```python
from build123d import *

# Parameters (mm, degrees)
F0_R     = 6.35
F1_DEPTH = 3.81


with BuildPart() as f1:
    # F0 (on Top) → F1 (new body, symmetric)
    with BuildSketch(Plane.XY):
        with BuildLine():
            Line((-22.269135, -16.838492), (-20.069431, -15.568492))
            ThreePointArc((-20.069431, -15.568492), (-17.960512, -17.960512), (-15.568492, -20.069431))
            Line((-15.568492, -20.069431), (-16.838492, -22.269135))
            Line((-16.838492, -22.269135), (-18.675675, -26.759218))
            Line((-18.675675, -26.759218), (-16.256, -28.156218))
            Line((-16.256, -28.156218), (-13.836325, -29.553218))
            Line((-13.836325, -29.553218), (-10.866391, -25.71713))
            Line((-10.866391, -25.71713), (-9.596391, -23.517425))
            ThreePointArc((-9.596391, -23.517425), (-6.574004, -24.534516), (-3.447994, -25.164883))
            Line((-3.447994, -25.164883), (-3.447994, -27.704883))
            Line((-3.447994, -27.704883), (-2.794, -32.512))
            Line((-2.794, -32.512), (0, -32.512))
            Line((0, -32.512), (2.794, -32.512))
            Line((2.794, -32.512), (3.447994, -27.704883))
            Line((3.447994, -27.704883), (3.447994, -25.164883))
            ThreePointArc((3.447994, -25.164883), (6.574004, -24.534516), (9.596391, -23.517425))
            Line((9.596391, -23.517425), (10.866391, -25.71713))
            Line((10.866391, -25.71713), (13.836325, -29.553218))
            Line((13.836325, -29.553218), (16.256, -28.156218))
            Line((16.256, -28.156218), (18.675675, -26.759218))
            Line((18.675675, -26.759218), (16.838492, -22.269135))
            Line((16.838492, -22.269135), (15.568492, -20.069431))
            ThreePointArc((15.568492, -20.069431), (17.960512, -17.960512), (20.069431, -15.568492))
            Line((20.069431, -15.568492), (22.269135, -16.838492))
            Line((22.269135, -16.838492), (26.759218, -18.675675))
            Line((26.759218, -18.675675), (28.156218, -16.256))
            Line((28.156218, -16.256), (29.553218, -13.836325))
            Line((29.553218, -13.836325), (25.71713, -10.866391))
            Line((25.71713, -10.866391), (23.517425, -9.596391))
            ThreePointArc((23.517425, -9.596391), (24.534516, -6.574004), (25.164883, -3.447994))
            ThreePointArc((25.164883, -3.447994), (25.4, 0), (25.164883, 3.447994))
            ThreePointArc((25.164883, 3.447994), (24.534516, 6.574004), (23.517425, 9.596391))
            ThreePointArc((23.517425, 9.596391), (21.997045, 12.7), (20.069431, 15.568492))
            ThreePointArc((20.069431, 15.568492), (17.960512, 17.960512), (15.568492, 20.069431))
            Line((15.568492, 20.069431), (16.838492, 22.269135))
            Line((16.838492, 22.269135), (18.675675, 26.759218))
            Line((18.675675, 26.759218), (16.256, 28.156218))
            Line((16.256, 28.156218), (13.836325, 29.553218))
            Line((13.836325, 29.553218), (10.866391, 25.71713))
            Line((10.866391, 25.71713), (9.596391, 23.517425))
            ThreePointArc((9.596391, 23.517425), (6.574004, 24.534516), (3.447994, 25.164883))
            Line((3.447994, 25.164883), (3.447994, 27.704883))
            Line((3.447994, 27.704883), (2.794, 32.512))
            Line((2.794, 32.512), (0, 32.512))
            Line((0, 32.512), (-2.794, 32.512))
            Line((-2.794, 32.512), (-3.447994, 27.704883))
            Line((-3.447994, 27.704883), (-3.447994, 25.164883))
            ThreePointArc((-3.447994, 25.164883), (-6.574004, 24.534516), (-9.596391, 23.517425))
            Line((-9.596391, 23.517425), (-10.866391, 25.71713))
            Line((-10.866391, 25.71713), (-13.836325, 29.553218))
            Line((-13.836325, 29.553218), (-16.256, 28.156218))
            Line((-16.256, 28.156218), (-18.675675, 26.759218))
            Line((-18.675675, 26.759218), (-16.838492, 22.269135))
            Line((-16.838492, 22.269135), (-15.568492, 20.069431))
            ThreePointArc((-15.568492, 20.069431), (-17.960512, 17.960512), (-20.069431, 15.568492))
            Line((-20.069431, 15.568492), (-22.269135, 16.838492))
            Line((-22.269135, 16.838492), (-26.759218, 18.675675))
            Line((-26.759218, 18.675675), (-28.156218, 16.256))
            Line((-28.156218, 16.256), (-29.553218, 13.836325))
            Line((-29.553218, 13.836325), (-25.71713, 10.866391))
            Line((-25.71713, 10.866391), (-23.517425, 9.596391))
            ThreePointArc((-23.517425, 9.596391), (-24.534516, 6.574004), (-25.164883, 3.447994))
            Line((-25.164883, 3.447994), (-27.704883, 3.447994))
            Line((-27.704883, 3.447994), (-32.512, 2.794))
            Line((-32.512, 2.794), (-32.512, 0))
            Line((-32.512, 0), (-32.512, -2.794))
            Line((-32.512, -2.794), (-27.704883, -3.447994))
            Line((-27.704883, -3.447994), (-25.164883, -3.447994))
            ThreePointArc((-25.164883, -3.447994), (-24.534516, -6.574004), (-23.517425, -9.596391))
            Line((-23.517425, -9.596391), (-25.71713, -10.866391))
            Line((-25.71713, -10.866391), (-29.553218, -13.836325))
            Line((-29.553218, -13.836325), (-28.156218, -16.256))
            Line((-28.156218, -16.256), (-26.759218, -18.675675))
            Line((-26.759218, -18.675675), (-22.269135, -16.838492))
        make_face()
        Circle(F0_R, mode=Mode.SUBTRACT)
    extrude(amount=F1_DEPTH, both=True)


solid = f1.part
```
Check sheet for the modelled part. Datum: model origin and axes. Units: mm. A direction names the side the tool comes from. Coordinates: 2 decimals unless noted, no trailing zeros. Order: outer loops, then holes, each group sorted by start corner. A loop starts at its lowest first (then second) coordinate and runs counter-clockwise, first axis right, second up. Notation, with made-up numbers: (84, 62.5) -> (139, 62.5) arc R20 cw to (139, 94.5) -> close; hole circle Ø10 at (41.5, 50.25). An arc over 180 degrees is marked (long way). Write item = value, one per line. Start each with the question number.
1) Cross-section at B-B (x = 0). Enter the section's corners in (y, z).
2) Cross-section at C-C (x = 7.5). Enter the section's corners in (y, z).
3) Cross-section at A-A (y = 0). Enter the section's corners in (x, z), then the cut area to 3 significant figures.
4) Access from +Z, -Z, +X, -X, +Y, -Y to the whole of each face (thin tool, end or side, straight path). Record for faces 1 (the flat face through (-3.126, -30.075, 0.053)), 2 (the cylindrical face through (24.546, 6.531, 0.053)), 3 (the flat face through (-24.6, -10.22, 0.05)), 4 (the flat face through (-32.512, 0, 0)), 5 (the flat face through (-10.22, 24.6, 0.05)).
5) Material ranges on L1, parallel to Y at x = 0, z = 1.25; L2, parallel to Y at x = -17.5, z = -1.5; L3, parallel to Y at x = -18.5, z = -2.5, recorded low to high.
6) Mould release check, pull along Y, two halves, no side actions. Record for faces 6 (the flat face through (-26, 3.448, 0)), 7 (the flat face through (3.116, -30.142, 0.053)), 8 (the flat face through (0, 32.512, 0)), 9 (the flat face through (-2, -7, -3.81)): +Y half, -Y half, draft (parallel to the pull), parting line (faces both ways), or undercut.
7) Go/stop test with flat-tipped pins: P1, Ø3, axis at x = -13.5, z = -1, coming from the +Y side; P2, Ø2, axis at y = -24, z = 1.5, coming from the +X side; P3, Ø0.8, axis at x = -26, z = 1.5, coming from the +Y side. Record where each tip stops, or that it passes through.
Ans:
q1.outline = (-32.51, -3.81) -> (-6.35, -3.81) -> (-6.35, 3.81) -> (-32.51, 3.81) -> close; (6.35, -3.81) -> (32.51, -3.81) -> (32.51, 3.81) -> (6.35, 3.81) -> close
q2.outline = (-24.27, -3.81) -> (24.27, -3.81) -> (24.27, 3.81) -> (-24.27, 3.81) -> close
q3.outline = (-32.51, -3.81) -> (-6.35, -3.81) -> (-6.35, 3.81) -> (-32.51, 3.81) -> close; (6.35, -3.81) -> (25.4, -3.81) -> (25.4, 3.81) -> (6.35, 3.81) -> close
q3.area = 345 mm²
q4.face_1 = +Z, -Z, -Y
q4.face_2 = +Z, -Z, +X, +Y
q4.face_3 = +Z, -Z, -X
q4.face_4 = +Z, -Z, -X, +Y, -Y
q4.face_5 = +Z, -Z, +Y
q5.L1 = -32.51 to -6.35, 6.35 to 32.51
q5.L2 = -27.44 to -23.89, -18.41 to 18.41, 23.89 to 27.44
q5.L3 = -26.86 to -26.33, -17.4 to 17.4, 26.33 to 26.86
q6.face_6 = undercut
q6.face_7 = -Y half
q6.face_8 = +Y half
q6.face_9 = draft
q7.P1 = 29.55
q7.P2 = 17.96
q7.P3 = 18.53
